For this review, take the finished solid that the model builds, in its own axes (mm). A direction names the side the tool comes from. Give positions to 0.01 mm unless a question says otherwise; leave off trailing zeros. Order: outer loops, then holes, each group sorted by start corner. A loop starts at its lowest first (then second) coordinate and runs counter-clockwise, first axis right, second up.
from build123d import *

# Parameters (mm, degrees)
BOSS_EXTRUDE1_DEPTH = 60
FILLET1_R           = 10
SKETCH2_R           = 4
CUT_EXTRUDE1_DEPTH  = 21
SKETCH3_R           = 6
SKETCH3_R_2         = 4
CUT_EXTRUDE2_DEPTH  = 10


with BuildPart() as part:
    # Sketch1 → Boss-Extrude1 (new body)
    with BuildSketch(Plane(origin=(0, 0, 0), x_dir=(1, 0, 0), z_dir=(0, 1, 0))):
        Polygon((-65, -5), (-100, -5), (-100, -25), (100, -25), (100, -5), (65, -5), (65, 25), (-65, 25), align=None)
    extrude(amount=BOSS_EXTRUDE1_DEPTH)

    # Fillet1
    fillet1_edges = [part.edges().sort_by_distance(p)[0] for p in [
        (-100, 0, 15),
        (-65, 30, 5),
        (-65, 30, -25),
        (65, 30, -25),
        (65, 30, 5),
        (-100, 60, 15),
        (100, 60, 15),
        (100, 0, 15),
    ]]
    fillet(fillet1_edges, radius=FILLET1_R)

    # Sketch2 → Cut-Extrude1 (cut, through all)
    with BuildSketch(Plane(origin=(0, 0, 5), x_dir=(-1, 0, 0), z_dir=(0, 0, -1))):
        with Locations((-88, 45)):
            Circle(SKETCH2_R)
        with Locations((-88, 15)):
            Circle(SKETCH2_R)
        with Locations((88, 15)):
            Circle(SKETCH2_R)
        with Locations((88, 45)):
            Circle(SKETCH2_R)
    extrude(amount=-CUT_EXTRUDE1_DEPTH, mode=Mode.SUBTRACT)

    # Sketch3 → Cut-Extrude2 (cut)
    with BuildSketch(Plane(origin=(0, 0, 5), x_dir=(-1, 0, 0), z_dir=(0, 0, -1))):
        with Locations((88, 15)):
            Circle(SKETCH3_R)
        with Locations((88, 15)):
            Circle(SKETCH3_R_2, mode=Mode.SUBTRACT)
        with Locations((88, 45)):
            Circle(SKETCH3_R)
        with Locations((88, 45)):
            Circle(SKETCH3_R_2, mode=Mode.SUBTRACT)
        with Locations((-88, 15)):
            Circle(SKETCH3_R)
        with Locations((-88, 15)):
            Circle(SKETCH3_R_2, mode=Mode.SUBTRACT)
        with Locations((-88, 45)):
            Circle(SKETCH3_R)
        with Locations((-88, 45)):
            Circle(SKETCH3_R_2, mode=Mode.SUBTRACT)
    extrude(amount=-CUT_EXTRUDE2_DEPTH, mode=Mode.SUBTRACT)


solid = part.part
1) We need section B-B on y = 15. Give the boundary of the cut face in (x, z).
Answer sheet:
outline: (-100, 5) - (-94, 5) - (-94, 15) - (-92, 15) - (-92, 25) - (-100, 25) - close; (-84, 15) - (-82, 15) - (-82, 5) - (-75, 5) arc R10 cw to (-65, -5) - (-65, -15) arc R10 ccw to (-55, -25) - (55, -25) arc R10 ccw to (65, -15) - (65, -5) arc R10 cw to (75, 5) - (82, 5) - (82, 15) - (84, 15) - (84, 25) - (-84, 25) - close; (92, 15) - (94, 15) - (94, 5) - (100, 5) - (100, 25) - (92, 25) - close
2) Tool access review of faces 1 (the face through (84.08, 16.42, 15)), 2 (the face through (88, 30, 5)), 3 (the face through (100, 30, 15)), 4 (the face through (-65, 30, -10)): name each direction out of +Z, -Z, +X, -X, +Y, -Y from which nothing blocks a thin tool from reaching the whole face with its end or side.
Answer sheet:
face 1: -Z
face 2: -Z, +X, +Y, -Y
face 3: +Z, -Z, +X, +Y, -Y
face 4: -Z, -X, +Y, -Y
3) Clearance check with flat-ended pins moving along their axes: pin 1 (14 mm diameter, centred on x = -88, y = 45, fed in from +Z); pin 2 (13 mm diameter, centred on x = -85.5, y = 13, fed in from -Z); pin 3 (3.5 mm diameter, centred on x = -88, y = 42.5, fed in from -Z); pin 4 (5 mm diameter, centred on y = 39.5, z = 1, fed in from +X). State where each tip first meets the part, or that it passes through.
Answer sheet:
pin 1: stops at z = 25
pin 2: stops at z = 5
pin 3: stops at z = 15
pin 4: stops at x = 69.73
4) To check wall thickness, follow line 1 (Y direction, x = -88, z = 20.75); line 2 (Y direction, x = 88, z = 8); line 3 (Z direction, x = -91, y = 29.5). State the ranges of each line that lie inside material, in increasing order.
Answer sheet:
line 1: y = 0 to 11, 19 to 41, 49 to 60
line 2: y = 0 to 9, 21 to 39, 51 to 60
line 3: z = 5 to 25
5) We need section C-C on z = -13. Give the boundary of the cut face in (x, y), then the cut area to 3 significant figures.
Answer sheet:
outline: (-65, 0) - (65, 0) - (65, 60) - (-65, 60) - close
area: 7,800 mm2
6) Draft analysis for pull direction X (two halves, no side actions). For faces 5 (the face through (-1, 0, 0)), 6 (the face through (84.305, 43.468, 19.93)), 7 (the face through (-68.01, 30.42, 2.15)), state which applies: +X half, -X half, draft (parallel to the pull), parting line (faces both ways), or undercut.
Answer sheet:
face 5: draft
face 6: undercut
face 7: -X half
7) We need section D-D on x = 62.5. Give the boundary of the cut face in (y, z).
Answer sheet:
outline: (0, -21.61) - (60, -21.61) - (60, 25) - (0, 25) - close
8) We need section A-A on x = 88. Give the boundary of the cut face in (y, z), then the cut area to 3 significant figures.
Answer sheet:
outline: (0, 5) - (9, 5) - (9, 15) - (11, 15) - (11, 25) - (0, 25) - close; (19, 15) - (21, 15) - (21, 5) - (39, 5) - (39, 15) - (41, 15) - (41, 25) - (19, 25) - close; (49, 15) - (51, 15) - (51, 5) - (60, 5) - (60, 25) - (49, 25) - close
area: 800 mm2
